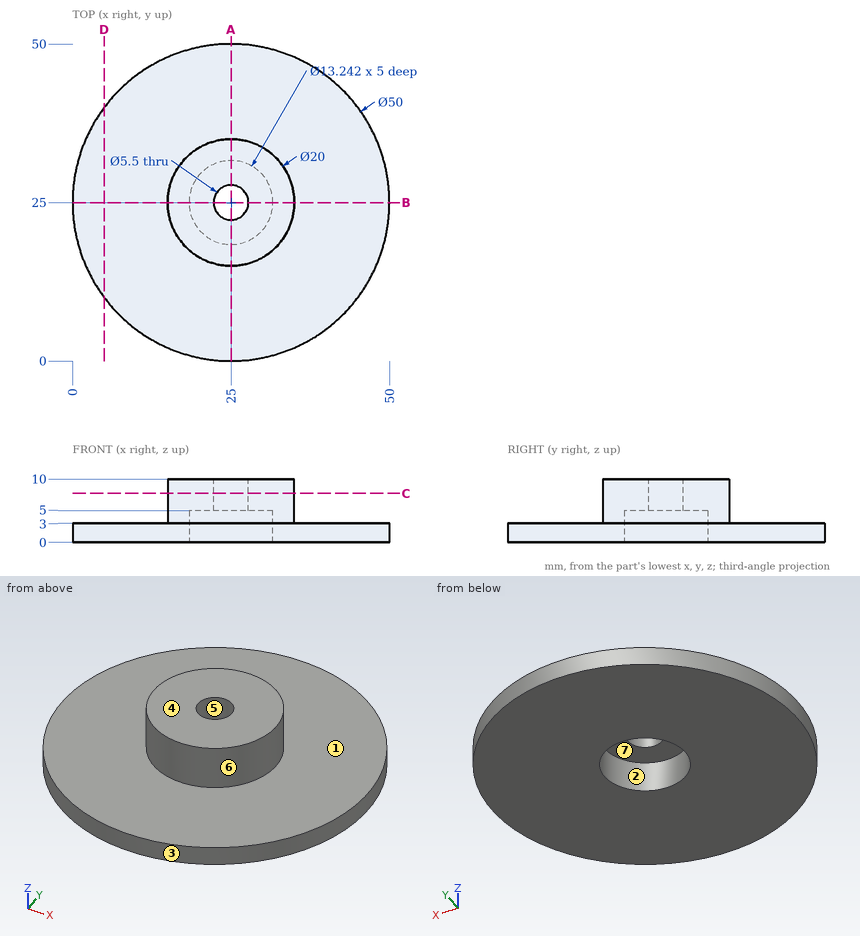
Drawing for the job (mm, zero at the part's lowest x, y, z). A direction names the side the tool comes from. Round coordinates to 2 decimals unless told otherwise and drop trailing zeros. Order: outer loops, then holes, each group sorted by start corner. A loop starts at its lowest first (then second) coordinate and runs counter-clockwise, first axis right, second up. Notation, with made-up numbers: M 50,-1 L 105,-1 A34 cw 105,32 Z; hole C 23,49.25 d1. An arc over 180 degrees is marked long. Use one line per item in the form item = value.
Q1. Two-plate mould, pull along X, no slides. Class the marked faces 4, 5, 6 and 7: +X half, -X half, draft (parallel to the pull), parting line (faces both ways), or undercut.
Recorded:
face_4 = draft
face_5 = undercut
face_6 = parting line
face_7 = undercut
Q2. Probe L1, parallel to Y at x = 25, z = 7.3; L2, parallel to Y at x = 25, z = 1.8. List the from-to ranges inside material, lowest first.
Recorded:
L1 = 15 to 22.25, 27.75 to 35
L2 = 0 to 18.38, 31.62 to 50
Q3. Saw through at A-A on x = 25. Give the cut face in (y, z), then the cut area to 3 significant figures.
Recorded:
outline = M 0,0 L 18.38,0 L 18.38,5 L 22.25,5 L 22.25,10 L 15,10 L 15,3 L 0,3 Z; M 27.75,5 L 31.62,5 L 31.62,0 L 50,0 L 50,3 L 35,3 L 35,10 L 27.75,10 Z
area = 196 mm^2
Q4. Saw through at C-C on z = 7.75. Give the cut face in (x, y), then the cut area to 3 significant figures.
Recorded:
outline = C 25,25 d20; hole C 25,25 d5.5
area = 290 mm^2
Q5. Which spindle directions (+Z, -Z, +X, -X, +Y, -Y) get a long thin tool onto all of the face, cutting with end or side? Do the marked faces 1, 2 and 3. Say none if no direction does.
Recorded:
face_1 = +Z
face_2 = -Z
face_3 = +Z, -Z
Q6. Saw through at D-D on x = 5. Give the cut face in (y, z), then the cut area to 3 significant figures.
Recorded:
outline = M 10,0 L 40,0 L 40,3 L 10,3 Z
area = 90.0 mm^2
Q7. Flat gauge pins, fed straight in: P1, Ø3, axis at y = 24, z = 5.5, coming from the -X side; P2, Ø6, axis at x = 37.5, z = 5.5, coming from the +Y side; P3, Ø5, axis at y = 35, z = 5, coming from the +X side. Where does each tip first touch, or does it go through?
Recorded:
P1 = 15
P2 = 47.53
P3 = 48.51
